Can you work these out from the model? Positions are in its coordinate system, mm. A direction names the side the tool comes from. Give positions to 0.01 mm unless a question says otherwise; leave off trailing zeros. Order: outer loops, then holes, each group sorted by start corner. A loop starts at its lowest first (then second) coordinate and runs counter-clockwise, first axis right, second up. Notation, with made-up numbers: (16.5, 70) - (32.5, 70) arc R21 cw to (32.5, 87) - close; hole circle Ø1 at (-0.5, 16). An arc over 180 degrees is marked (long way). Return JSON: item names as keys, results as strings.
```python
from build123d import *

# Parameters (mm, degrees)
CUT_EXTRUDE2_START = -45.15
CUT_EXTRUDE2_DEPTH = 18.85


with BuildPart() as part:
    # Sketch1 → Revolve1 (revolve)
    with BuildSketch(Plane.XY, mode=Mode.PRIVATE) as revolve1_sk:
        Polygon((0, 0), (-45.15, 0), (-45.15, 3.9), (-25.6, 3.9), (-25.6, 3.75), (-24.9, 3.75), (-24.9, 4), (-20, 4), (-20, 5), (-13, 5), (-13, 4), (-8.1, 4), (-8.1, 3.75), (-7.4, 3.75), (-7.4, 3.9), (0, 3.9), align=None)
    revolve(revolve1_sk.sketch.rotate(Axis((0, 0, 0), (-1, 0, 0)), 90), axis=Axis((0, 0, 0), (-1, 0, 0)))

    # Sketch2 → Cut-Extrude2 (cut)
    with BuildSketch(Plane(origin=(0, 0, 0), x_dir=(0, 0, -1), z_dir=(1, 0, 0)).offset(CUT_EXTRUDE2_START)):
        with BuildLine():
            Line((2, -3.348133809), (-2, -3.348133809))
            ThreePointArc((-2, -3.348133809), (0, -3.9), (2, -3.348133809))
        make_face()
    extrude(amount=CUT_EXTRUDE2_DEPTH, mode=Mode.SUBTRACT)


solid = part.part
```
1. Suppose I cut it at C-C (x = -10). List the corners of the cut face in (y, z) for me.
Checks:
{"outline": "circle Ø8 at (0, 0)"}
2. On a 3-axis mill with a long thin cutter (end or side, diameter ignored), from which of +Z, -Z, +X, -X, +Y, -Y can I reach the whole of each face in a straight line? I mean faces 1 (the face through (-25.25, -3.16, -2.02)), 2 (the face through (-3.65, -2.64, 2.87)), 3 (the face through (-35.238, 3.807, 0.845)), 4 (the face through (-36, -3.348, 0)). Say none if no direction works.
Checks:
{"face 1": "none", "face 2": "+X", "face 3": "-X", "face 4": "+Z, -Z, -X, -Y"}
3. For pin 1 Ø4 at (x, y) = (-34.5, -3.5) entering from +Z; pin 2 Ø4 at (x, y) = (-17, -3) entering from +Z; pin 3 Ø3 at (x, z) = (-24, -0.5) entering from -Y, each with a flat end and sliding along its axis, tell me the tip position at first contact or that it passes through.
Checks:
{"pin 1": "z = 3.6", "pin 2": "z = 4.9", "pin 3": "y = -4"}
4. If I drill on L1, parallel to X at y = -3.5, z = 1.5; L2, parallel to X at y = -4, z = 0.5; L3, parallel to Y at x = -29.5, z = -1.75, over which ranges is the centre line in solid material (lowest first)? Write a range as [from, to].
Checks:
{"L1": "[-26.3, -25.6], [-24.9, -8.1], [-7.4, 0]", "L2": "[-20, -13]", "L3": "[-3.35, 3.49]"}
5. Suppose I cut it at A-A (y = 0). List the corners of the cut face in (x, z) for me, plus the area to 3 significant figures.
Checks:
{"outline": "(-45.15, -3.9) - (-25.6, -3.9) - (-25.6, -3.75) - (-24.9, -3.75) - (-24.9, -4) - (-20, -4) - (-20, -5) - (-13, -5) - (-13, -4) - (-8.1, -4) - (-8.1, -3.75) - (-7.4, -3.75) - (-7.4, -3.9) - (0, -3.9) - (0, 3.9) - (-7.4, 3.9) - (-7.4, 3.75) - (-8.1, 3.75) - (-8.1, 4) - (-13, 4) - (-13, 5) - (-20, 5) - (-20, 4) - (-24.9, 4) - (-24.9, 3.75) - (-25.6, 3.75) - (-25.6, 3.9) - (-45.15, 3.9) - close", "area": "369 mm^2"}
6. Suppose I cut it at D-D (y = 3.25). List the corners of the cut face in (x, z) for me, plus the area to 3 significant figures.
Checks:
{"outline": "(-45.15, -2.16) - (-25.6, -2.16) - (-25.6, -1.87) - (-24.9, -1.87) - (-24.9, -2.33) - (-20, -2.33) - (-20, -3.8) - (-13, -3.8) - (-13, -2.33) - (-8.1, -2.33) - (-8.1, -1.87) - (-7.4, -1.87) - (-7.4, -2.16) - (0, -2.16) - (0, 2.16) - (-7.4, 2.16) - (-7.4, 1.87) - (-8.1, 1.87) - (-8.1, 2.33) - (-13, 2.33) - (-13, 3.8) - (-20, 3.8) - (-20, 2.33) - (-24.9, 2.33) - (-24.9, 1.87) - (-25.6, 1.87) - (-25.6, 2.16) - (-45.15, 2.16) - close", "area": "220 mm^2"}
